Autodesk Inventor part; units mm, degrees
ref_plane "YZ Plane" through (0, 0, 0) normal (1, 0, 0) x (0, 1, 0)
ref_plane "XZ Plane" through (0, 0, 0) normal (0, 1, 0) x (-1, 0, 0)
ref_plane "XY Plane" through (0, 0, 0) normal (0, 0, 1) x (1, 0, 0)
sketch "Sketch1" plane through (0, 0, 0) normal (0, 0, 1) x (1, 0, 0)
  line L0 (0, 0) -> (-284.4922, 0)
  line L1 (0, 0) -> (0, 292.5)
  line L2 (0, 292.5) -> (-52.4, 292.5)
  line L3 (-52.4, 292.5) -> (-52.4, 212.5)
  line L4 (-52.4, 212.5) -> (-54.4, 212.5)
  line L5 (-54.4, 212.5) -> (-54.4, 0)
  dimension "d0" = 585
  dimension "d1" = 52.4
  dimension "d2" = 2
  dimension "d3" = 425
revolve "Revolution1" add sketch "Sketch1" angle 360 about axis through (0, 0, 0) along (-1, 0, 0)
sketch "Sketch2" plane through (0, 0, 0) normal (1, 0, 0) x (0, 0, -1)
  point P0 (0, 0)
  point P1 (0, 257.2)
  dimension "d5" = 257.2
hole "Hole1" at (0, 257.2, 0) direction (-1, 0, 0) diameter 31.75 end up to surface
pattern_circular "Circular Pattern1" count 20 over 360 about axis through (-26.2, 0, 0) along (1, 0, 0) of "Hole1"
properties part number "Blind Flange 14 in" material "ASTM A105 Gr.B"
Verification items for the finished model (mm, model axes). A direction names the side the tool comes from. Coordinates: 2 decimals unless noted, no trailing zeros. Loops run counter-clockwise (first coordinate to the right, second up) from the corner with the lowest first, then second, coordinate; pieces in that order, holes last. Notation, with made-up numbers: (-40, 83.5) - (17, 83.5) arc R23 ccw to (17, 105.5) - close; hole circle Ø3 at (28.5, 0). An arc over 180 degrees is marked (long way). Answer as a JSON object with one key per item and string values.
(1) Cross-section at B-B, the plane x = -23. Count the separate pieces of the cut face and the enclosed holes in it, then the cut area to 3 significant figures.
Response:
{"separate pieces": "1", "enclosed holes": "20", "area": "253,000 mm²"}
(2) Scan lines: line 1 along Z through (x, y) = (-32.5, 0) (3 decimals); line 2 along Z through (x, y) = (-3, -197.5); line 3 along Y through (x, z) = (-9.5, 238.5). Record each from-to range of solid material in increasing order.
Response:
{"line 1": "z = -292.5 to -273.075, -241.325 to 241.325, 273.075 to 292.5", "line 2": "z = -215.75 to -163.01, -139.34 to 139.34, 163.01 to 215.75", "line 3": "y = -169.33 to -94.13, -64.83 to 64.83, 94.13 to 169.33"}
(3) Go/stop test with flat-tipped pins: pin 1 Ø6 at (x, y) = (-21, -85.5) entering from +Z; pin 2 Ø19 at (y, z) = (151.18, -208.08) entering from -X; pin 3 Ø12 at (x, z) = (-35, -192.5) entering from -Y; pin 4 Ø12 at (y, z) = (-173, 174.5) entering from -X. Record where each tip stops, or that it passes through.
Response:
{"pin 1": "stops at z = 280.62", "pin 2": "passes through", "pin 3": "stops at y = -225.33", "pin 4": "stops at x = -52.4"}
(4) Mould release check, pull along Z, two halves, no side actions. Record for faces 3 (the cylindrical face through (-26.567, 278.993, -87.859)), 4 (the flat face through (-52.4, -153, -153)), 5 (the cylindrical face through (-26.57, 68.75, -232.91)): pulls with the +Z half, pulls with the -Z half, needs draft (parallel to the pull), parting line crosses it, or undercut.
Response:
{"face 3": "parting line crosses it", "face 4": "needs draft", "face 5": "undercut"}
(5) Cross-section at A-A, the plane z = 0. Record the boundary of the cut face in (x, y) (3 decimals).
Response:
{"outline": "(-54.4, -212.5) - (-52.4, -212.5) - (-52.4, -241.325) - (0, -241.325) - (0, 241.325) - (-52.4, 241.325) - (-52.4, 212.5) - (-54.4, 212.5) - close; (-52.4, -292.5) - (0, -292.5) - (0, -273.075) - (-52.4, -273.075) - close; (-52.4, 273.075) - (0, 273.075) - (0, 292.5) - (-52.4, 292.5) - close"}
(6) Access from +Z, -Z, +X, -X, +Y, -Y to the whole of each face (thin tool, end or side, straight path). Record for faces 1 (the cylindrical face through (-26.567, 222.163, -158.504)), 2 (the cylindrical face through (-53.414, -27.663, -210.692)).
Response:
{"face 1": "+X, -X", "face 2": "-X"}
(7) Cross-section at C-C, the plane z = -116.5. Record the boundary of the cut face in (x, y), then the cut area to 3 significant figures.
Response:
{"outline": "(-54.4, -177.72) - (-52.4, -177.72) - (-52.4, -268.3) - (0, -268.3) - (0, 268.3) - (-52.4, 268.3) - (-52.4, 177.72) - (-54.4, 177.72) - close", "area": "28,800 mm²"}
